Design review of the part built by this model. Coordinates are the model's own, in mm. Round coordinates to 2 decimals unless told otherwise and drop trailing zeros. Loops run counter-clockwise (first coordinate to the right, second up) from the corner with the lowest first, then second, coordinate; pieces in that order, holes last. Notation, with made-up numbers: (84, 52.25) - (93, 52.25) arc R10 cw to (93, 70.25) - close; hole circle Ø6 at (48.25, -20.75). An arc over 180 degrees is marked (long way). One line per question, with ' | ' between items. Start each with the question number.
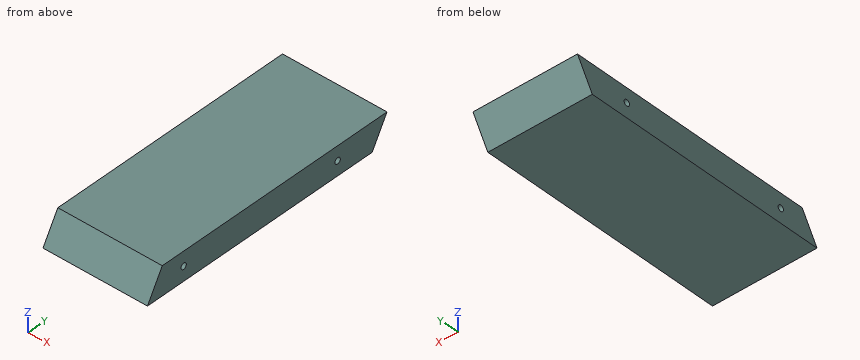
from build123d import *

# Parameters (mm, degrees)
F0_W          = 139.7
F0_H          = 38.1
F1_DEPTH      = 177.8
F1_DEPTH_BACK = 177.8
F3_DEPTH      = 139.7
F4_R          = 3.96875
F5_DEPTH      = 139.701


with BuildPart() as f1:
    # F0 (on Front) → F1 (new body, two sides)
    with BuildSketch(Plane.XZ) as f1_sk:
        Rectangle(F0_W, F0_H)
    extrude(amount=F1_DEPTH)
    extrude(f1_sk.sketch, amount=-F1_DEPTH_BACK)

    # F2 (on face) → F3 (cut, through all)
    with BuildSketch(Plane(origin=(-69.85, 0, 0), x_dir=(0, -1, 0), z_dir=(-1, 0, 0))):
        Polygon((-155.802955, -19.05), (-177.8, 19.05), (-177.8, -19.05), align=None)
        Polygon((177.8, -19.05), (177.8, 19.05), (155.802955, 19.05), align=None)
    extrude(amount=-F3_DEPTH, mode=Mode.SUBTRACT)

    # F4 (on face) → F5 (cut, through all)
    with BuildSketch(Plane(origin=(-69.85, 0, 0), x_dir=(0, -1, 0), z_dir=(-1, 0, 0))):
        with Locations((-104.547045, 0)):
            Circle(F4_R)
        with Locations((124.052955, 0)):
            Circle(F4_R)
    extrude(amount=-F5_DEPTH, mode=Mode.SUBTRACT)


solid = f1.part
1. Clearance check with flat-ended pins moving along their axes: P1, Ø1, axis at x = 6.5, z = -1, coming from the +Y side; P2, Ø10.5, axis at y = -124.05, z = 0, coming from the +X side; P3, Ø4, axis at x = 42, z = -5, coming from the -Y side; P4, Ø1.5, axis at x = -35.5, z = -4.5, coming from the -Y side. State where each tip first meets the part, or that it passes through.
2. Take a section at B-B, the plane z = 0. Give the boundary of the cut face in (x, y), then the cut area to 3 significant figures.
3. Take a section at A-A, the plane x = 2. Give the boundary of the cut face in (y, z).
4. To check wall thickness, follow line 1 along Y through (x, z) = (14.5, 1); line 2 along Z through (x, y) = (-40.5, 106); line 3 along Y through (x, z) = (54, -14). State the ranges of each line that lie inside material, in increasing order.
Answer list:
1) P1: stops at y = 166.51 | P2: stops at x = 69.85 | P3: stops at y = -170.84 | P4: stops at y = -169.83
2) outline: (-69.85, -166.8) - (69.85, -166.8) - (69.85, -128.02) - (-69.85, -128.02) - close; (-69.85, -120.08) - (69.85, -120.08) - (69.85, 100.58) - (-69.85, 100.58) - close; (-69.85, 108.52) - (69.85, 108.52) - (69.85, 166.8) - (-69.85, 166.8) - close | area: 44,400 mm²
3) outline: (-177.8, -19.05) - (155.8, -19.05) - (177.8, 19.05) - (-155.8, 19.05) - close; hole circle Ø7.94 at (-124.05, 0); hole circle Ø7.94 at (104.55, 0)
4) line 1: y = -166.22 to -127.89, -120.21 to 100.71, 108.39 to 167.38 | line 2: z = -19.05 to -3.69, 3.69 to 19.05 | line 3: y = -174.88 to 158.72
